The model under review builds one solid part; all positions refer to its coordinate system, in mm. Give positions to 0.01 mm unless a question says otherwise; leave off trailing zeros. Write each loop counter-clockwise with the first axis right and the second up, starting at its lowest first coordinate (ties: lowest second). Pieces come first, ordered by that corner, then holes.
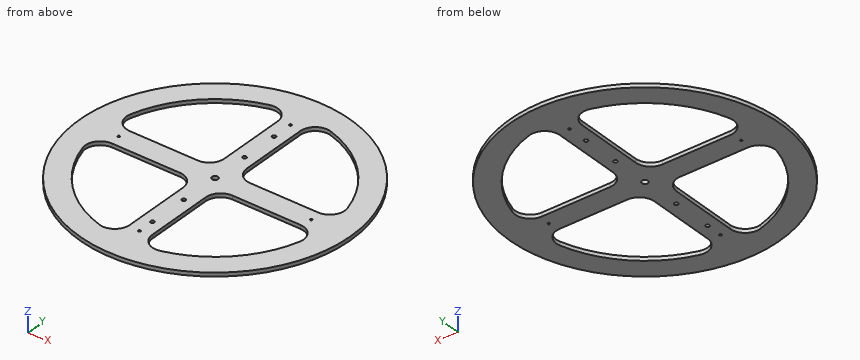
from build123d import *

# Parameters (mm, degrees)
SKETCH1_R           = 180
BOSS_EXTRUDE1_DEPTH = 5
SKETCH2_R           = 4
CUT_EXTRUDE1_DEPTH  = 6
SKETCH3_R           = 2.5
CUT_EXTRUDE2_DEPTH  = 6
SKETCH4_R           = 1.5
CUT_EXTRUDE3_DEPTH  = 6


with BuildPart() as part:
    # Sketch1 → Boss-Extrude1 (new body)
    with BuildSketch(Plane.XY):
        Circle(SKETCH1_R)
        with BuildLine():
            Line((-15, 125.199840255), (-15, 35))
            ThreePointArc((-15, 35), (-20.857864376, 20.857864376), (-35, 15))
            Line((-35, 15), (-125.199840255, 15))
            ThreePointArc((-125.199840255, 15), (-141.132390392, 22.910589503), (-144.461354141, 40.384615385))
            ThreePointArc((-144.461354141, 40.384615385), (-106.066017178, 106.066017178), (-40.384615385, 144.461354141))
            ThreePointArc((-40.384615385, 144.461354141), (-22.910589503, 141.132390392), (-15, 125.199840255))
        make_face(mode=Mode.SUBTRACT)
        with BuildLine():
            Line((15, 125.199840255), (15, 35))
            ThreePointArc((15, 35), (20.857864376, 20.857864376), (35, 15))
            Line((35, 15), (125.199840255, 15))
            ThreePointArc((125.199840255, 15), (141.132390392, 22.910589503), (144.461354141, 40.384615385))
            ThreePointArc((144.461354141, 40.384615385), (106.066017178, 106.066017178), (40.384615385, 144.461354141))
            ThreePointArc((40.384615385, 144.461354141), (22.910589503, 141.132390392), (15, 125.199840255))
        make_face(mode=Mode.SUBTRACT)
        with BuildLine():
            Line((125.199840255, -15), (35, -15))
            ThreePointArc((35, -15), (20.857864376, -20.857864376), (15, -35))
            Line((15, -35), (15, -125.199840255))
            ThreePointArc((15, -125.199840255), (22.910589503, -141.132390392), (40.384615385, -144.461354141))
            ThreePointArc((40.384615385, -144.461354141), (106.066017178, -106.066017178), (144.461354141, -40.384615385))
            ThreePointArc((144.461354141, -40.384615385), (141.132390392, -22.910589503), (125.199840255, -15))
        make_face(mode=Mode.SUBTRACT)
        with BuildLine():
            Line((-15, -35), (-15, -125.199840255))
            ThreePointArc((-15, -125.199840255), (-22.910589503, -141.132390392), (-40.384615385, -144.461354141))
            ThreePointArc((-40.384615385, -144.461354141), (-106.066017178, -106.066017178), (-144.461354141, -40.384615385))
            ThreePointArc((-144.461354141, -40.384615385), (-141.132390392, -22.910589503), (-125.199840255, -15))
            Line((-125.199840255, -15), (-35, -15))
            ThreePointArc((-35, -15), (-20.857864376, -20.857864376), (-15, -35))
        make_face(mode=Mode.SUBTRACT)
    extrude(amount=BOSS_EXTRUDE1_DEPTH)

    # Sketch2 → Cut-Extrude1 (cut, through all)
    with BuildSketch(Plane.XY.offset(5)):
        Circle(SKETCH2_R)
    extrude(amount=-CUT_EXTRUDE1_DEPTH, mode=Mode.SUBTRACT)

    # Sketch3 → Cut-Extrude2 (cut, through all)
    with BuildSketch(Plane.XY.offset(5)):
        with Locations((0, 50)):
            Circle(SKETCH3_R)
        with Locations((0, 100)):
            Circle(SKETCH3_R)
        with Locations((0, -53)):
            Circle(SKETCH3_R)
        with Locations((0, -106)):
            Circle(SKETCH3_R)
    extrude(amount=-CUT_EXTRUDE2_DEPTH, mode=Mode.SUBTRACT)

    # Sketch4 → Cut-Extrude3 (cut, through all)
    with BuildSketch(Plane.XY.offset(5)):
        with Locations((0, 128)):
            Circle(SKETCH4_R)
        with Locations((128, 0)):
            Circle(SKETCH4_R)
        with Locations((0, -128)):
            Circle(SKETCH4_R)
        with Locations((-128, 0)):
            Circle(SKETCH4_R)
    extrude(amount=-CUT_EXTRUDE3_DEPTH, mode=Mode.SUBTRACT)


solid = part.part
1) Consider section B-B, the plane z = 1.35. State how many separate pieces and enclosed holes the cut face has, then the cut area to 3 significant figures.
2) To check wall thickness, follow probe 1 along X at (y, z) = (-96.5, 3.9); probe 2 along X at (y, z) = (-127, 4.6); probe 3 along Y at (x, z) = (128, 3.95). State the ranges of each line that lie inside material, in increasing order.
3) Consider section A-A, the plane x = -85.5. Give the boundary of the cut face in (y, z), then the cut area to 3 significant figures.
4) Insertion check: pin 1 (5 mm diameter, centred on x = 0, y = -128, fed in from -Z); pin 2 (1 mm diameter, centred on y = -79, z = 2, fed in from +X); pin 3 (1.5 mm diameter, centred on x = 70.5, z = 2.5, fed in from +Y); pin 4 (2.5 mm diameter, centred on x = 84.5, z = 2.5, fed in from -Y). Each pin has a flat end and moves straight along its axis. Give the tip position at first contact, or say it passes through.
Answer block:
1. separate pieces: 1
1. enclosed holes: 13
1. area: 49,500 mm2
2. probe 1: x = -151.95 to -114.84, -15 to 15, 114.84 to 151.95
2. probe 2: x = -127.56 to -79.82, -15.08 to -1.12, 1.12 to 15.08, 79.82 to 127.56
2. probe 3: y = -126.55 to -78.2, -15.2 to -1.5, 1.5 to 15.2, 78.2 to 126.55
3. outline: (-158.4, 0) - (-123.25, 0) - (-123.25, 5) - (-158.4, 5) - close; (-15, 0) - (15, 0) - (15, 5) - (-15, 5) - close; (123.25, 0) - (158.4, 0) - (158.4, 5) - (123.25, 5) - close
3. area: 502 mm2
4. pin 1: stops at z = 0
4. pin 2: stops at x = 161.98
4. pin 3: stops at y = 165.94
4. pin 4: stops at y = -159.59
